Source: CAD feature listing. Evaluate the final solid. Frame: model axes, mm. A direction names the side the tool comes from. Round coordinates to 2 decimals unless told otherwise and drop trailing zeros. Order: outer loops, then holes, each group sorted by start corner. A loop starts at its lowest first (then second) coordinate and runs counter-clockwise, first axis right, second up. Notation, with made-up numbers: (-25.75, 5) -> (11.25, 5) arc R12 cw to (11.25, 19) -> close; hole circle Ø2 at (42.25, 3.5). An arc over 180 degrees is marked (long way). One line per item, written item: value. Start each with the question number.
1) Section C-C (y = 1). Return the cut outline in (x, z), and give its area (3 significant figures).
2) Ray query, L1, parallel to X at y = 3.25, z = 32.5; L2, parallel to X at y = 4.75, z = 13.5; L3, parallel to X at y = 1, z = -21.5. Return the intervals inside material, ascending.
3) Pin query (flat end, axial travel): P1, Ø5, axis at x = -29, y = 7, coming from the -Z side; P2, Ø2.5, axis at x = 12.79, z = -27.51, coming from the -Y side; P3, Ø4, axis at x = 7.5, z = 9, coming from the -Y side; P4, Ø5, axis at y = 6, z = -13, coming from the -X side. Return the tip coordinate at first contact, or that it passes through.
4) Mould query, pull axis Z, two halves, no side actions, for faces 4 (the face through (-19.711, 5, 19)), 5 (the face through (-37.145, 4.93, 30.993)), 6 (the face through (10, 5, -30.508)). Classes: pulls with the +Z half, pulls with the -Z half, needs draft (parallel to the pull), parting line crosses it, or undercut.
5) Section B-B (x = -7). Return the cut outline in (y, z), and give its area (3 significant figures).
6) Reachability of faces 1 (the face through (-30, 5, 9.492)), 2 (the face through (12.855, 4.93, 30.993)), 3 (the face through (5.289, 5, 0)) from +Z, -Z, +X, -X, +Y, -Y: full face, straight path, thin tool, end or side. Return the list, or none.
7) Section A-A (z = 16.5). Return the cut outline in (x, y).
8) Section D-D (z = 6.5). Return the cut outline in (x, y).
```python
from build123d import *

# Parameters (mm, degrees)
ESQUISSE1_R        = 1.5
BOSS_EXTRU_1_DEPTH = 10


with BuildPart() as part:
    # Esquisse1 → Boss.-Extru.1 (new body)
    with BuildSketch(Plane(origin=(0, 0, 0), x_dir=(1, 0, 0), z_dir=(0, 1, 0))):
        Polygon((5.288808664, 30.508122744), (15.288808664, 30.508122744), (15.288808664, -35.491877256), (-39.711191336, -35.491877256), (-39.711191336, -9.491877256), (-19.711191336, -9.491877256), (-19.711191336, -29.491877256), (5.288808664, -29.491877256), align=None)
        with Locations(Location((12.788808664, -32.491877256, 0), (0, 0, 270))):
            Circle(ESQUISSE1_R, mode=Mode.SUBTRACT)
        with Locations(Location((-37.211191336, -32.491877256, 0), (0, 0, 270))):
            Circle(ESQUISSE1_R, mode=Mode.SUBTRACT)
        with Locations(Location((12.788808664, 27.508122744, 0), (0, 0, 270))):
            Circle(ESQUISSE1_R, mode=Mode.SUBTRACT)
    extrude(amount=BOSS_EXTRU_1_DEPTH)


solid = part.part
```
Findings:
1. outline: (-39.71, 9.49) -> (-19.71, 9.49) -> (-19.71, 29.49) -> (5.29, 29.49) -> (5.29, -30.51) -> (15.29, -30.51) -> (15.29, 35.49) -> (-39.71, 35.49) -> close; hole circle Ø3 at (-37.21, 32.49); hole circle Ø3 at (12.79, -27.51); hole circle Ø3 at (12.79, 32.49)
1. area: 1,310 mm2
2. L1: -39.71 to -38.71, -35.71 to 11.29, 14.29 to 15.29
2. L2: -39.71 to -19.71, 5.29 to 15.29
2. L3: 5.29 to 15.29
3. P1: z = 9.49
3. P2: through
3. P3: y = 0
3. P4: x = 5.29
4. face 4: needs draft
4. face 5: undercut
4. face 6: pulls with the -Z half
5. outline: (0, 29.49) -> (10, 29.49) -> (10, 35.49) -> (0, 35.49) -> close
5. area: 60.0 mm2
6. face 1: -Z, -X, +Y, -Y
6. face 2: +Y, -Y
6. face 3: -Z, +Y, -Y
7. outline: (-39.71, 0) -> (-19.71, 0) -> (-19.71, 10) -> (-39.71, 10) -> close; (5.29, 0) -> (15.29, 0) -> (15.29, 10) -> (5.29, 10) -> close
8. outline: (5.29, 0) -> (15.29, 0) -> (15.29, 10) -> (5.29, 10) -> close
